from build123d import *

# Parameters (mm, degrees)
F0_W      = 75
F0_H      = 60
F1_DEPTH  = 36
F2_R      = 2
F3_R      = 2
F4_R      = 2
F5_R      = 2
F6_R      = 2
F7_T      = -2.25
F8_R      = 2.5
F9_DEPTH  = 27
F10_W     = 13
F10_H     = 8.5
F11_DEPTH = 25
F12_R     = 1.5
F13_DEPTH = 25


with BuildPart() as f1:
    # F0 (on Top) → F1 (new body)
    with BuildSketch(Plane.XY):
        Rectangle(F0_W, F0_H)
    extrude(amount=F1_DEPTH)

    # F2
    f2_edges = [f1.edges().sort_by_distance(p)[0] for p in [
        (-37.5, 30, 18),
    ]]
    fillet(f2_edges, radius=F2_R)

    # F3
    f3_edges = [f1.edges().sort_by_distance(p)[0] for p in [
        (37.5, 30, 18),
    ]]
    fillet(f3_edges, radius=F3_R)

    # F4
    f4_edges = [f1.edges().sort_by_distance(p)[0] for p in [
        (37.5, -30, 18),
    ]]
    fillet(f4_edges, radius=F4_R)

    # F5
    f5_edges = [f1.edges().sort_by_distance(p)[0] for p in [
        (-37.5, -30, 18),
    ]]
    fillet(f5_edges, radius=F5_R)

    # F6
    f6_edges = [f1.edges().sort_by_distance(p)[0] for p in [
        (37.5, 0, 36),
        (0, -30, 36),
        (-37.5, 0, 36),
        (-36.914214, -29.414214, 36),
        (36.914214, -29.414214, 36),
        (-36.914214, 29.414214, 36),
        (36.914214, 29.414214, 36),
        (0, 30, 36),
    ]]
    fillet(f6_edges, radius=F6_R)

    # F7
    f7_openings = [f1.faces().sort_by_distance(p)[0] for p in [
        (0, 0, 0),
    ]]
    offset(amount=F7_T, openings=f7_openings)

    # F8 (on face) → F9 (join)
    with BuildSketch(Plane(origin=(0, 0, 33.75), x_dir=(1, 0, 0), z_dir=(0, 0, -1))):
        with Locations((-32.636665, 0)):
            Circle(F8_R)
        with Locations((32.640941, 0)):
            Circle(F8_R)
    extrude(amount=F9_DEPTH)

    # F10 (on face) → F11 (cut)
    with BuildSketch(Plane(origin=(-37.5, 0, 0), x_dir=(0, -1, 0), z_dir=(-1, 0, 0))):
        with Locations((14.25, 27.55)):
            Rectangle(F10_W, F10_H)
    extrude(amount=-F11_DEPTH, mode=Mode.SUBTRACT)

    # F12 (on face) → F13 (cut)
    with BuildSketch(Plane.XY.offset(36)):
        with Locations((-17.2, 16.2)):
            Circle(F12_R)
    extrude(amount=-F13_DEPTH, mode=Mode.SUBTRACT)


solid = f1.part
CAD build for the part. Positions are in the model's coordinates, mm. A direction names the side the tool comes from. Coordinates: 2 decimals unless noted, no trailing zeros. Loops run counter-clockwise (first coordinate to the right, second up) from the corner with the lowest first, then second, coordinate; pieces in that order, holes last. Notation, with made-up numbers: (88, 22) -> (139, 22) arc R14 cw to (139, 41) -> close; hole circle Ø6 at (34, 5.25). An arc over 180 degrees is marked (long way). One line per item, written item: value.
1. Pull direction Z, two halves, no side cores. Call faces 4 (the face through (33, 0, 6.75)), 5 (the face through (0, -27.75, 17)), 6 (the face through (-36, -20.75, 27)): pulls with the +Z half, pulls with the -Z half, needs draft (parallel to the pull), parting line crosses it, or undercut.
Answers:
face 4: pulls with the -Z half
face 5: needs draft
face 6: undercut
2. Slice it at B-B on z = 20.5. Write the cut outline in (x, y), and give its area (3 significant figures).
Answers:
outline: (-37.5, -28) arc R2 ccw to (-35.5, -30) -> (35.5, -30) arc R2 ccw to (37.5, -28) -> (37.5, 28) arc R2 ccw to (35.5, 30) -> (-35.5, 30) arc R2 ccw to (-37.5, 28) -> close; circle Ø5 at (-32.64, 0); circle Ø5 at (32.64, 0); hole (-35.25, -27.75) -> (35.25, -27.75) -> (35.25, 27.75) -> (-35.25, 27.75) -> close
area: 623 mm^2
3. Which spindle directions (+Z, -Z, +X, -X, +Y, -Y) get a long thin tool onto all of the face, cutting with end or side? Do faces 1 (the face through (-0.5, 29.43, 35.4)), 2 (the face through (-33, 0, 6.75)), 3 (the face through (-36, -14, 31.8)). Say none if no direction does.
Answers:
face 1: +Z, +X, -X, +Y
face 2: -Z
face 3: -X
4. Slice it at A-A on y = -16. Write the cut outline in (x, z), and give its area (3 significant figures).
Answers:
outline: (-37.5, 0) -> (-35.25, 0) -> (-35.25, 23.3) -> (-37.5, 23.3) -> close; (-37.5, 31.8) -> (-35.25, 31.8) -> (-35.25, 33.75) -> (35.25, 33.75) -> (35.25, 0) -> (37.5, 0) -> (37.5, 34) arc R2 ccw to (35.5, 36) -> (-35.5, 36) arc R2 ccw to (-37.5, 34) -> close
area: 300 mm^2
5. Slice it at D-D on z = 4.5. Write the cut outline in (x, y).
Answers:
outline: (-37.5, -28) arc R2 ccw to (-35.5, -30) -> (35.5, -30) arc R2 ccw to (37.5, -28) -> (37.5, 28) arc R2 ccw to (35.5, 30) -> (-35.5, 30) arc R2 ccw to (-37.5, 28) -> close; hole (-35.25, -27.75) -> (35.25, -27.75) -> (35.25, 27.75) -> (-35.25, 27.75) -> close
6. Flat gauge pins, fed straight in: P1, Ø8, axis at x = -26.5, y = 21, coming from the -Z side; P2, Ø0.7, axis at x = -37, z = 29.5, coming from the -Y side; P3, Ø4, axis at x = -32, y = -1, coming from the -Z side. Where does each tip first touch, or does it go through?
Answers:
P1: stops at z = 33.75
P2: stops at y = -29.64
P3: stops at z = 6.75
7. Slice it at C-C on x = -17.2. Write the cut outline in (y, z), and give its area (3 significant figures).
Answers:
outline: (-30, 0) -> (-27.75, 0) -> (-27.75, 33.75) -> (14.7, 33.75) -> (14.7, 36) -> (-28, 36) arc R2 ccw to (-30, 34) -> close; (17.7, 33.75) -> (27.75, 33.75) -> (27.75, 0) -> (30, 0) -> (30, 34) arc R2 ccw to (28, 36) -> (17.7, 36) -> close
area: 278 mm^2
8. Drill centre lines: line 1 (Y direction, x = -15, z = 26); line 2 (X direction, y = -12.5, z = 16.5); line 3 (X direction, y = 16, z = 34). Where is each one in solid material? Low to high. Write a range as [from, to].
Answers:
line 1: y = [-30, -27.75], [27.75, 30]
line 2: x = [-37.5, -35.25], [35.25, 37.5]
line 3: x = [-37.5, -18.69], [-15.71, 37.5]
